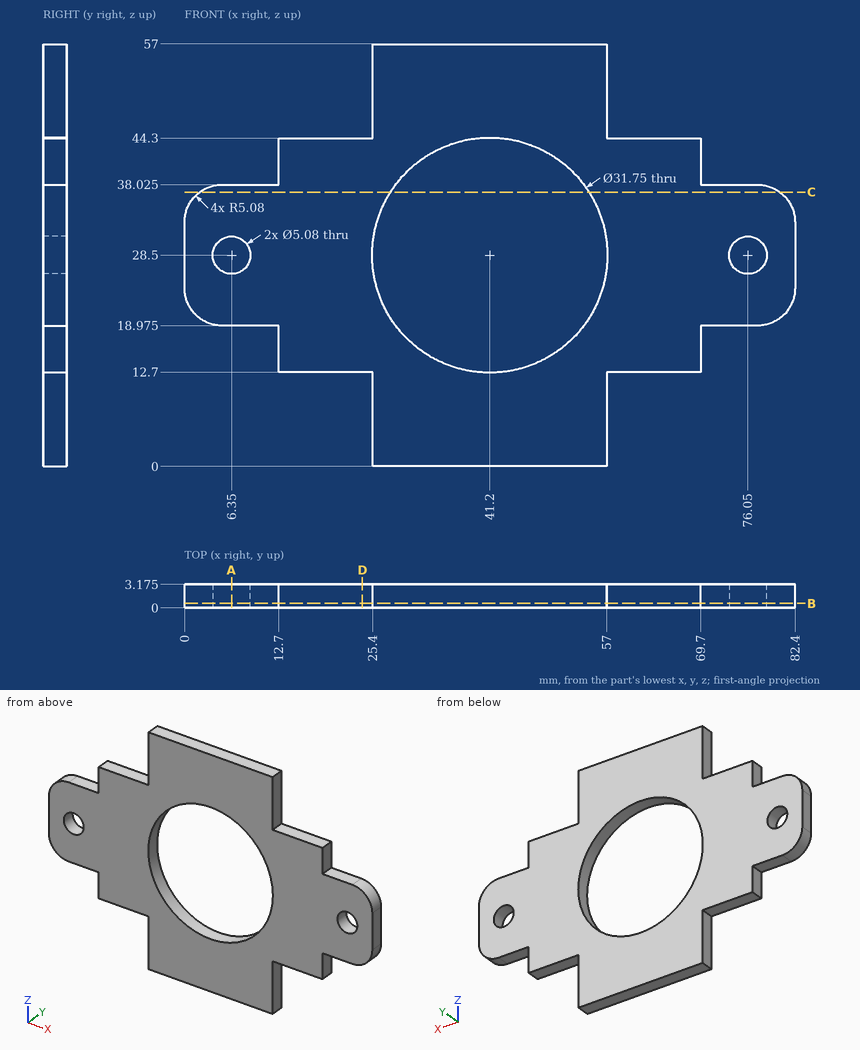
Input: dimensioned drawing with shaded views. Units: mm. Origin: part minimum x, y, z. Round coordinates to 2 decimals unless told otherwise and drop trailing zeros. Loops run counter-clockwise (first coordinate to the right, second up) from the corner with the lowest first, then second, coordinate; pieces in that order, holes last.
1) Section query C-C on z = 37. Return the cut outline in (x, y) (3 decimals).
Ans:
outline: (2.02, 0) - (27.792, 0) - (27.792, 3.175) - (2.02, 3.175) - close; (54.608, 0) - (80.38, 0) - (80.38, 3.175) - (54.608, 3.175) - close
2) Section query D-D on x = 24. Return the cut outline in (y, z) (3 decimals).
Ans:
outline: (0, 12.7) - (3.175, 12.7) - (3.175, 44.3) - (0, 44.3) - close
3) Material intervals for line 1 (Z direction, x = 6.35, y = 1.4) (3 decimals); line 2 (X direction, y = 1.9, z = 28); line 3 (X direction, y = 2.5, z = 9), sorted ascending.
Ans:
line 1: z = 18.975 to 25.96, 31.04 to 38.025
line 2: x = 0 to 3.86, 8.84 to 25.33, 57.07 to 73.56, 78.54 to 82.4
line 3: x = 25.4 to 57
4) Section query B-B on y = 0.6. Return the cut outline in (x, z) (3 decimals), plus the area to 3 significant figures.
Ans:
outline: (0, 24.055) arc R5.08 ccw to (5.08, 18.975) - (12.7, 18.975) - (12.7, 12.7) - (25.4, 12.7) - (25.4, 0) - (57, 0) - (57, 12.7) - (69.7, 12.7) - (69.7, 18.975) - (77.32, 18.975) arc R5.08 ccw to (82.4, 24.055) - (82.4, 32.945) arc R5.08 ccw to (77.32, 38.025) - (69.7, 38.025) - (69.7, 44.3) - (57, 44.3) - (57, 57) - (25.4, 57) - (25.4, 44.3) - (12.7, 44.3) - (12.7, 38.025) - (5.08, 38.025) arc R5.08 ccw to (0, 32.945) - close; hole circle Ø5.08 at (6.35, 28.5); hole circle Ø31.75 at (41.2, 28.5); hole circle Ø5.08 at (76.05, 28.5)
area: 2,230 mm2
5) Pin query (flat end, axial travel): pin 1 (6.5 mm diameter, centred on x = 76.05, z = 28.5, fed in from +Y) (3 decimals); pin 2 (1.6 mm diameter, centred on x = 9.5, y = 2, fed in from -Z) (3 decimals); pin 3 (1 mm diameter, centred on y = 1, z = 4, fed in from -X); pin 4 (1 mm diameter, centred on x = 7.5, y = 2, fed in from +Z) (3 decimals). Return the tip coordinate at first contact, or that it passes through.
Ans:
pin 1: stops at y = 3.175
pin 2: stops at z = 18.975
pin 3: stops at x = 25.4
pin 4: stops at z = 38.025
6) Section query A-A on x = 6.35. Return the cut outline in (y, z) (3 decimals).
Ans:
outline: (0, 18.975) - (3.175, 18.975) - (3.175, 25.96) - (0, 25.96) - close; (0, 31.04) - (3.175, 31.04) - (3.175, 38.025) - (0, 38.025) - close
